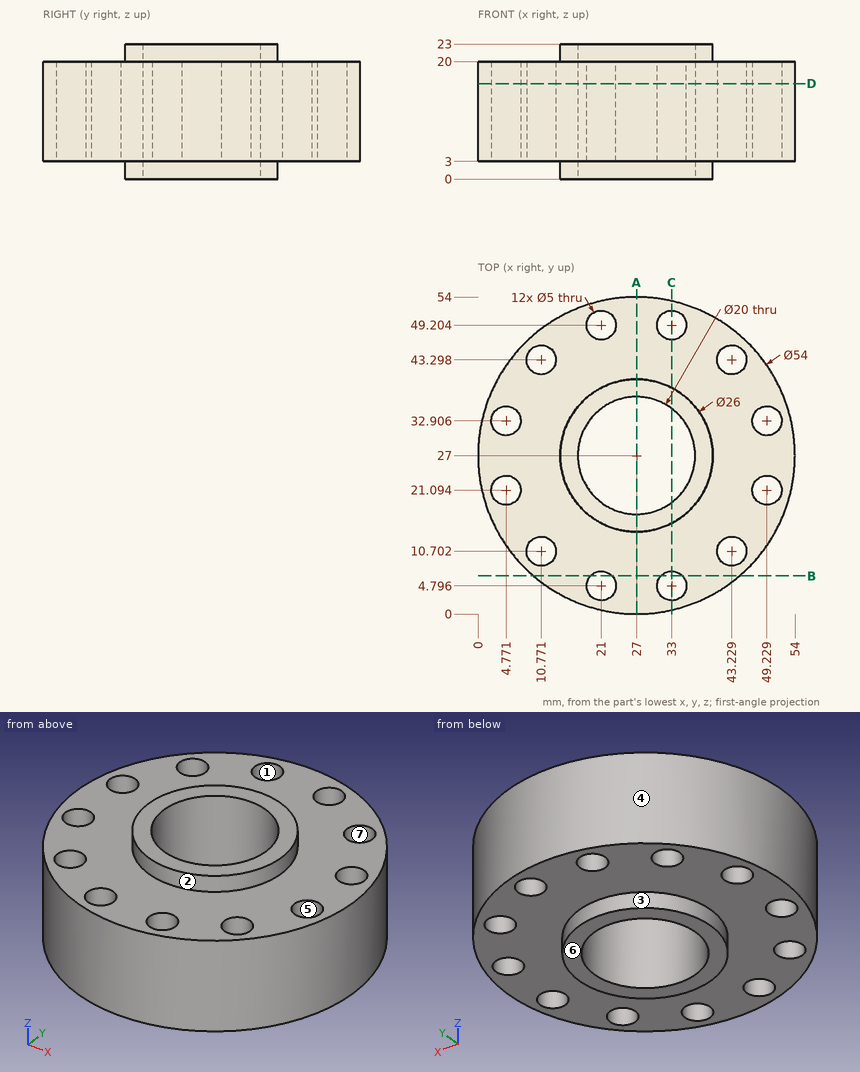
Geometry check sheet. Reference: drawing and pictorial views, mm from the part's lowest x, y, z. A direction names the side the tool comes from. Round coordinates to 2 decimals unless told otherwise and drop trailing zeros. Write each loop counter-clockwise with the first axis right and the second up, starting at its lowest first coordinate (ties: lowest second). Pieces come first, ordered by that corner, then holes.
1. Gauge pin test, flat ends, axial feed: P1, Ø8, axis at x = 33.5, y = 8.5, coming from the +Z side; P2, Ø6, axis at x = 14.5, z = 3.5, coming from the -Y side; P3, Ø6.5, axis at x = 49.23, y = 32.91, coming from the -Z side. Record the tip position at first contact, or that the pin passes through.
2. Section check D-D on z = 16.25. State how many separate pieces and enclosed holes the cut face has, plus the area to 3 significant figures.
3. Section check C-C on x = 33. Enter the section's corners in (y, z) (1 decimal).
4. Access from +Z, -Z, +X, -X, +Y, -Y to the whole of each face (thin tool, end or side, straight path). Record for the marked faces 1, 2 and 3.
5. Section check A-A on x = 27. Enter the section's corners in (y, z).
6. Section check B-B on y = 6.5. Enter the section's corners in (x, z).
7. Draft check along X on the marked faces 4, 5, 6 and 7. Enter one of: +X half, -X half, draft (parallel to the pull), parting line (faces both ways), or undercut.
8. Scan lines: L1, parallel to X at y = 41, z = 7 (1 decimal); L2, parallel to X at y = 42.5, z = 11; L3, parallel to X at y = 32, z = 19.5. Record each from-to range of solid material in increasing order.
Answer:
1. P1: stops at z = 20
1. P2: stops at y = 1.73
1. P3: stops at z = 3
2. separate pieces: 1
2. enclosed holes: 13
2. area: 1,740 mm2
3. outline: (0.7, 3) - (2.3, 3) - (2.3, 20) - (0.7, 20) - close; (7.3, 3) - (15.5, 3) - (15.5, 0) - (19, 0) - (19, 23) - (15.5, 23) - (15.5, 20) - (7.3, 20) - close; (35, 0) - (38.5, 0) - (38.5, 3) - (46.7, 3) - (46.7, 20) - (38.5, 20) - (38.5, 23) - (35, 23) - close; (51.7, 3) - (53.3, 3) - (53.3, 20) - (51.7, 20) - close
4. face 1: +Z, -Z
4. face 2: +Z
4. face 3: -Z
5. outline: (0, 3) - (14, 3) - (14, 0) - (17, 0) - (17, 23) - (14, 23) - (14, 20) - (0, 20) - close; (37, 0) - (40, 0) - (40, 3) - (54, 3) - (54, 20) - (40, 20) - (40, 23) - (37, 23) - close
6. outline: (9.43, 3) - (19.17, 3) - (19.17, 20) - (9.43, 20) - close; (22.83, 3) - (31.17, 3) - (31.17, 20) - (22.83, 20) - close; (34.83, 3) - (44.57, 3) - (44.57, 20) - (34.83, 20) - close
7. face 4: parting line
7. face 5: undercut
7. face 6: draft
7. face 7: undercut
8. L1: x = 3.9 to 9.8, 11.8 to 42.2, 44.2 to 50.1
8. L2: x = 4.89 to 8.4, 13.14 to 40.86, 45.6 to 49.11
8. L3: x = 0.47 to 2.44, 7.1 to 18.34, 35.66 to 46.9, 51.56 to 53.53
